```python
from build123d import *

# Parameters (mm, degrees)
ESQUISSE1_R        = 50
ESQUISSE1_R_2      = 1.6
BOSS_EXTRU_1_DEPTH = 2


with BuildPart() as part:
    # Esquisse1 → Boss.-Extru.1 (new body)
    with BuildSketch(Plane(origin=(0, 0, 0), x_dir=(1, 0, 0), z_dir=(0, 1, 0))):
        with Locations(Location((0, 0, 0), (0, 0, 270))):
            Circle(ESQUISSE1_R)
        with Locations(Location((-30, 30, 0), (0, 0, 270))):
            Circle(ESQUISSE1_R_2, mode=Mode.SUBTRACT)
        with Locations(Location((30, 30, 0), (0, 0, 90))):
            Circle(ESQUISSE1_R_2, mode=Mode.SUBTRACT)
        with Locations(Location((30, -30, 0), (0, 0, 270))):
            Circle(ESQUISSE1_R_2, mode=Mode.SUBTRACT)
        with Locations(Location((-30, -30, 0), (0, 0, 90))):
            Circle(ESQUISSE1_R_2, mode=Mode.SUBTRACT)
    extrude(amount=BOSS_EXTRU_1_DEPTH)


solid = part.part
```
Input: part model. Units: mm. Frame: model coordinates. Give positions to 0.01 mm unless a question says otherwise; leave off trailing zeros. Order: outer loops, then holes, each group sorted by start corner. A loop starts at its lowest first (then second) coordinate and runs counter-clockwise, first axis right, second up.
1. Mould query, pull axis Z, two halves, no side actions, for faces 1 (the cylindrical face through (15.02, 0.99, 47.69)), 2 (the cylindrical face through (-31.08, 0.99, 31.18)), 3 (the flat face through (1, 2, -1)). Classes: released by +Z, released by -Z, zero draft, split by the parting line, or undercut.
Derived:
face 1: split by the parting line
face 2: undercut
face 3: zero draft
2. Section C-C on y = 1.2. Return the cut outline in (x, z).
Derived:
outline: circle Ø100 at (0, 0); hole circle Ø3.2 at (-30, -30); hole circle Ø3.2 at (-30, 30); hole circle Ø3.2 at (30, -30); hole circle Ø3.2 at (30, 30)
3. Material intervals for L1, parallel to X at y = 0.75, z = 30; L2, parallel to X at y = 0.7, z = 1; L3, parallel to X at y = 0.5, z = -29.5, sorted ascending.
Derived:
L1: x = -40 to -31.6, -28.4 to 28.4, 31.6 to 40
L2: x = -49.99 to 49.99
L3: x = -40.37 to -31.52, -28.48 to 28.48, 31.52 to 40.37
4. Pin query (flat end, axial travel): pin 1 (4 mm diameter, centred on x = -33.5, z = 0, fed in from -Y); pin 2 (1 mm diameter, centred on x = -18, y = 1.5, fed in from +Z). Return the tip coordinate at first contact, or that it passes through.
Derived:
pin 1: stops at y = 0
pin 2: stops at z = 46.84
5. Section A-A on x = -30. Return the cut outline in (y, z).
Derived:
outline: (0, -40) - (2, -40) - (2, -31.6) - (0, -31.6) - close; (0, -28.4) - (2, -28.4) - (2, 28.4) - (0, 28.4) - close; (0, 31.6) - (2, 31.6) - (2, 40) - (0, 40) - close
6. Section B-B on z = 30. Return the cut outline in (x, y).
Derived:
outline: (-40, 0) - (-31.6, 0) - (-31.6, 2) - (-40, 2) - close; (-28.4, 0) - (28.4, 0) - (28.4, 2) - (-28.4, 2) - close; (31.6, 0) - (40, 0) - (40, 2) - (31.6, 2) - close
7. Section D-D on z = 40. Return the cut outline in (x, y).
Derived:
outline: (-30, 0) - (30, 0) - (30, 2) - (-30, 2) - close
